from build123d import *

# Parameters (mm, degrees)
BOSS_EXTRUDE1_DEPTH = 76.2


with BuildPart() as part:
    # Sketch1 → Boss-Extrude1 (new body)
    with BuildSketch(Plane.XY):
        with BuildLine():
            Line((-11, 0), (-13.54, 0))
            ThreePointArc((-13.54, 0), (-12.046376905, 6.181941723), (-7.895036415, 11))
            Line((-7.895036415, 11), (-27.94, 11))
            Line((-27.94, 11), (-27.94, 13.54))
            Line((-27.94, 13.54), (27.94, 13.54))
            Line((27.94, 13.54), (27.94, 11))
            Line((27.94, 11), (7.895036415, 11))
            ThreePointArc((7.895036415, 11), (12.046376905, 6.181941723), (13.54, 0))
            Line((13.54, 0), (11, 0))
            ThreePointArc((11, 0), (0, 11), (-11, 0))
        make_face()
    extrude(amount=BOSS_EXTRUDE1_DEPTH)


solid = part.part
Build history of the part. All positions in model axes, mm. A direction names the side the tool comes from. Coordinates: 2 decimals unless noted, no trailing zeros. Write each loop counter-clockwise with the first axis right and the second up, starting at its lowest first coordinate (ties: lowest second). Pieces come first, ordered by that corner, then holes.
(1) Pin check, flat tips, straight feed: pin 1 Ø10 at (x, z) = (-22.5, 31.5) entering from -Y; pin 2 Ø2 at (y, z) = (8, 9.5) entering from -X. Stop position of each tip, or through.
(2) Drill centre lines: line 1 (Y direction, x = 19, z = 35); line 2 (X direction, y = 5.25, z = 59); line 3 (X direction, y = 9, z = 53.5). Where is each one in solid material? Low to high.
(3) Mould opens along Y. For faces 3 (the flat face through (-18, 11, 38)), 4 (the cylindrical face through (-12.09, 6.1, 37.57)), 5 (the flat face through (-27.94, 12, 38)), 6 (the cylindrical face through (0, 11, 38)) say: pulls with the +Y half, pulls with the -Y half, needs draft (parallel to the pull), parting line crosses it, or undercut.
(4) Cut at A-A on z = 34. List the corners of the cut face in (x, y).
(5) Cut at C-C on x = 0. List the corners of the cut face in (y, z).
(6) Cut at B-B on y = 1.75. List the corners of the cut face in (x, z), and give its area (3 significant figures).
(7) 3-axis set-ups, long thin cutter, end or side, ignore diameter. For faces 1 (the flat face through (27.94, 12, 38)), 2 (the flat face through (18, 11, 38)): which of +Z, -Z, +X, -X, +Y, -Y reach the whole face in a straight line?
(8) Cut at D-D on x = 7. List the corners of the cut face in (y, z), and give its area (3 significant figures).
Working result:
1. pin 1: stops at y = 11
1. pin 2: stops at x = -11.59
2. line 1: y = 11 to 13.54
2. line 2: x = -12.48 to -9.67, 9.67 to 12.48
2. line 3: x = -10.12 to -6.32, 6.32 to 10.12
3. face 3: undercut
3. face 4: undercut
3. face 5: needs draft
3. face 6: pulls with the -Y half
4. outline: (-27.94, 11) - (-7.9, 11) arc R13.54 ccw to (-13.54, 0) - (-11, 0) arc R11 cw to (11, 0) - (13.54, 0) arc R13.54 ccw to (7.9, 11) - (27.94, 11) - (27.94, 13.54) - (-27.94, 13.54) - close
5. outline: (11, 0) - (13.54, 0) - (13.54, 76.2) - (11, 76.2) - close
6. outline: (-13.43, 0) - (-10.86, 0) - (-10.86, 76.2) - (-13.43, 76.2) - close; (10.86, 0) - (13.43, 0) - (13.43, 76.2) - (10.86, 76.2) - close
6. area: 391 mm2
7. face 1: +Z, -Z, +X, +Y, -Y
7. face 2: +Z, -Z, +X
8. outline: (8.49, 0) - (13.54, 0) - (13.54, 76.2) - (8.49, 76.2) - close
8. area: 385 mm2
